from build123d import *

# Parameters (mm, degrees)
SKETCH1_W           = 76.2
SKETCH1_H           = 63.5
BOSS_EXTRUDE1_DEPTH = 6.35
SKETCH2_W           = 76.2
SKETCH2_H           = 6.35
BOSS_EXTRUDE2_DEPTH = 50.8
SKETCH3_R           = 3.175
BOSS_EXTRUDE3_DEPTH = 25.4


with BuildPart() as part:
    # Sketch1 → Boss-Extrude1 (new body)
    with BuildSketch(Plane(origin=(0, 0, 0), x_dir=(1, 0, 0), z_dir=(0, 1, 0))):
        Rectangle(SKETCH1_W, SKETCH1_H)
    extrude(amount=BOSS_EXTRUDE1_DEPTH)

    # Sketch2 → Boss-Extrude2 (add)
    with BuildSketch(Plane(origin=(0, 6.35, 0), x_dir=(1, 0, 0), z_dir=(0, 1, 0))):
        with Locations((0, 28.575)):
            Rectangle(SKETCH2_W, SKETCH2_H)
        with Locations((0, -28.575)):
            Rectangle(SKETCH2_W, SKETCH2_H)
    extrude(amount=BOSS_EXTRUDE2_DEPTH)

    # Sketch3 → Boss-Extrude3 (add)
    with BuildSketch(Plane.XZ):
        with Locations(Location((0, 0, 0), (0, 0, 270))):
            Circle(SKETCH3_R)
    extrude(amount=BOSS_EXTRUDE3_DEPTH)


solid = part.part
Here's how the part is built. I have some questions about the finished solid (model axes, mm). A direction names the side the tool comes from. Coordinates: 2 decimals unless noted, no trailing zeros. Order: outer loops, then holes, each group sorted by start corner. A loop starts at its lowest first (then second) coordinate and runs counter-clockwise, first axis right, second up.
Item 1: I need wall thicknesses on line 1 (Z direction, x = 6.5, y = 28); line 2 (Y direction, x = -31, z = 6); line 3 (Y direction, x = -6.5, z = 28). Which ranges of each line are inside material? Lowest first, please.
Result sheet:
line 1: z = -31.75 to -25.4, 25.4 to 31.75
line 2: y = 0 to 6.35
line 3: y = 0 to 57.15
Item 2: If we mould it in two halves opening along Z, with no side actions, what happens to faces 1 (the face through (-1, 6.35, 0)), 2 (the face through (38.1, 5, 3)), 3 (the face through (-1, 31, 25.4)), 4 (the face through (-1, 28, -31.75))? For each: +Z half, -Z half, draft (parallel to the pull), parting line (faces both ways), or undercut.
Result sheet:
face 1: undercut
face 2: draft
face 3: undercut
face 4: -Z half
Item 3: If we section it at B-B on x = 15: List the corners of the cut face in (y, z) for me.
Result sheet:
outline: (0, -31.75) - (57.15, -31.75) - (57.15, -25.4) - (6.35, -25.4) - (6.35, 25.4) - (57.15, 25.4) - (57.15, 31.75) - (0, 31.75) - close
Item 4: If we section it at D-D on x = 0: List the corners of the cut face in (y, z) for me (3 decimals).
Result sheet:
outline: (-25.4, -3.175) - (0, -3.175) - (0, -31.75) - (57.15, -31.75) - (57.15, -25.4) - (6.35, -25.4) - (6.35, 25.4) - (57.15, 25.4) - (57.15, 31.75) - (0, 31.75) - (0, 3.175) - (-25.4, 3.175) - close
Item 5: If we section it at A-A on y = 7.5: List the corners of the cut face in (x, z) for me, plus the area to 3 significant figures.
Result sheet:
outline: (-38.1, -31.75) - (38.1, -31.75) - (38.1, -25.4) - (-38.1, -25.4) - close; (-38.1, 25.4) - (38.1, 25.4) - (38.1, 31.75) - (-38.1, 31.75) - close
area: 968 mm2
Item 6: If we section it at C-C on z = 0: List the corners of the cut face in (x, y) for me (3 decimals).
Result sheet:
outline: (-38.1, 0) - (-3.175, 0) - (-3.175, -25.4) - (3.175, -25.4) - (3.175, 0) - (38.1, 0) - (38.1, 6.35) - (-38.1, 6.35) - close
Item 7: For faces 5 (the face through (-1.93, -12.52, 2.52)), 6 (the face through (-1, 31, -25.4)), 7 (the face through (-1, 57.15, -29)), which set-ups out of +Z, -Z, +X, -X, +Y, -Y let a thin tool reach every point of the face, with its end or its side?
Result sheet:
face 5: -Y
face 6: +X, -X, +Y
face 7: +Z, -Z, +X, -X, +Y
Item 8: For P1, Ø8, axis at x = -20.5, z = 12, coming from the +Y side; P2, Ø12, axis at x = 28, z = -20, coming from the -Y side, each with a flat end and sliding along its axis, tell me the tip position at first contact or that it passes through.
Result sheet:
P1: stops at y = 6.35
P2: stops at y = 0
